Job drawing, mm, ordinate dimensions from the low corner. One solid piece. Give positions to 0.01 mm unless a question says otherwise; leave off trailing zeros. Write each loop counter-clockwise with the first axis right and the second up, starting at its lowest first coordinate (ties: lowest second). Pieces come first, ordered by that corner, then holes. Notation, with made-up numbers: (73.5, 66) -> (119.5, 66) arc R9 cw to (119.5, 70) -> close; hole circle Ø4 at (-18.75, -12.75). An arc over 180 degrees is marked (long way). One line per question, with ' | ' between items. Start each with the question number.
(1) Pull direction X, two halves, no side cores. Call the marked faces 1, 2 and 3: released by +X, released by -X, zero draft, split by the parting line, or undercut.
(2) Drill centre lines: probe 1 along Y at (x, z) = (5, 7.5); probe 2 along X at (y, z) = (7.5, 7.75); probe 3 along Y at (x, z) = (1.75, 6.5). Where is each one in solid material? Low to high. Write a range as from..to.
(3) Band-saw the part on C-C, the plane z = 21.75. Give the cut face in (x, y).
(4) Band-saw the part on B-B, the plane x = 5. Give the cut face in (y, z), and give its area (3 significant figures).
(5) Pin check, flat tips, straight feed: P1, Ø3, axis at y = 1.5, z = 10.5, coming from the -X side; P2, Ø5, axis at x = 1.5, z = 7.5, coming from the +Y side. Stop position of each tip, or through.
(6) Band-saw the part on A-A, the plane y = 5. Give the cut face in (x, z), and give its area (3 significant figures).
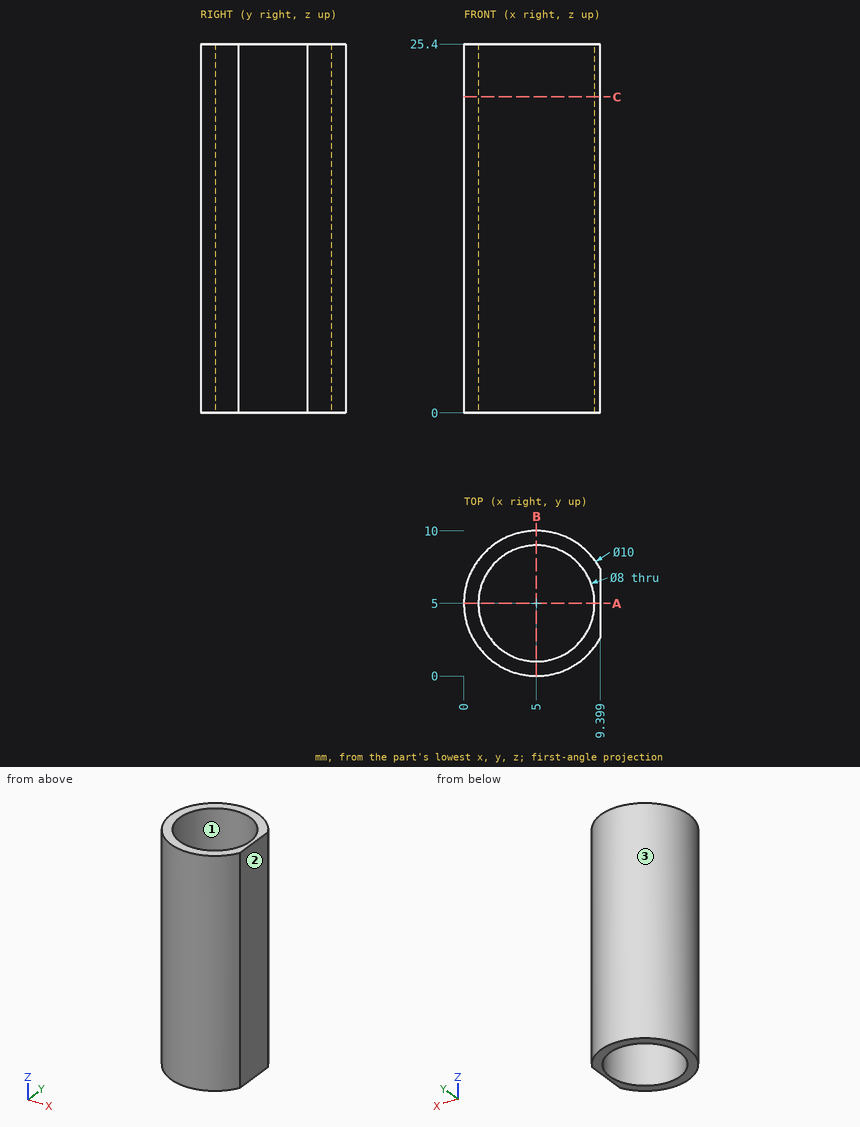
Results:
1) face 1: undercut | face 2: released by +X | face 3: split by the parting line
2) probe 1: y = 0..1, 9..10 | probe 2: x = 0.67..1.88, 8.12..9.33 | probe 3: y = 1.2..2.67, 7.33..8.8
3) outline: (9.4, 2.62) -> (9.4, 7.38) arc R5 ccw (long way) to start; hole circle Ø8 at (5, 5)
4) outline: (0, 0) -> (1, 0) -> (1, 25.4) -> (0, 25.4) -> close; (9, 0) -> (10, 0) -> (10, 25.4) -> (9, 25.4) -> close | area: 50.8 mm²
5) P1: stops at x = 0.42 | P2: stops at y = 9.9
6) outline: (0, 0) -> (1, 0) -> (1, 25.4) -> (0, 25.4) -> close; (9, 0) -> (9.4, 0) -> (9.4, 25.4) -> (9, 25.4) -> close | area: 35.5 mm²
